Autodesk Inventor part; units mm, degrees
ref_plane "YZ Plane" through (0, 0, 0) normal (1, 0, 0) x (0, 1, 0)
ref_plane "XZ Plane" through (0, 0, 0) normal (0, 1, 0) x (-1, 0, 0)
ref_plane "XY Plane" through (0, 0, 0) normal (0, 0, 1) x (1, 0, 0)
sketch "Sketch1" plane through (0, 0, 0) normal (0, 1, 0) x (-1, 0, 0)
  line L0 (120, 102) -> (90, 102)
  line L1 (120, -102) -> (90, -102)
  line L2 (120, 102) -> (120, -102)
  line L3 (90, 102) -> (90, 50)
  line L4 (90, -50) -> (90, -102)
  line L5 (90, 50) -> (15, 50)
  line L6 (90, -50) -> (15, -50)
  line L7 (15, 50) -> (15, 102)
  line L8 (15, -50) -> (15, -102)
  line L9 (15, 102) -> (-15, 102)
  line L10 (15, -102) -> (-15, -102)
  line L11 (-15, 102) -> (-15, 50)
  line L12 (-15, -50) -> (-15, -102)
  line L13 (-15, 50) -> (-90, 50)
  line L14 (-15, -50) -> (-90, -50)
  line L15 (-90, 50) -> (-90, 102)
  line L16 (-90, -50) -> (-90, -102)
  line L17 (-90, 102) -> (-120, 102)
  line L18 (-90, -102) -> (-120, -102)
  line L19 (-120, 102) -> (-120, -102)
  line L20 (120, 0) -> (-120, 0) construction
  line L21 (0, 102) -> (0, -102) construction
  point P0 (0, 0)
  point P1 (0, 0)
  dimension "d0" = 204
  dimension "d1" = 30
  dimension "d3" = 75
  dimension "d4" = 52
  dimension "d5" = 100
extrude "Extrusion1" add sketch "Sketch1" along normal blind 5
sketch "Sketch2" plane through (0, 5, 0) normal (0, 1, 0) x (1, 0, 0)
  line L0 (-115, -90.5) -> (-95, -90.5)
  line L1 (-95, -90.5) -> (-95, -50)
  line L2 (-95, -50) -> (-115, -50)
  line L3 (-115, -50) -> (-115, -90.5)
  line L4 (-120, -102) -> (-90, -102)
  line L5 (-120, 102) -> (-120, -102)
  line L6 (-90, -102) -> (-90, -50)
  line L7 (-10, -90.5) -> (10, -90.5)
  line L8 (10, -90.5) -> (10, -50)
  line L9 (10, -50) -> (-10, -50)
  line L10 (-10, -50) -> (-10, -90.5)
  line L11 (95, -90.5) -> (115, -90.5)
  line L12 (115, -90.5) -> (115, -50)
  line L13 (115, -50) -> (95, -50)
  line L14 (95, -50) -> (95, -90.5)
  line L15 (-15, -50) -> (-15, -102)
  line L16 (90, -50) -> (90, -102)
  line L17 (-115, 50) -> (-95, 50)
  line L18 (-95, 50) -> (-95, 90.5)
  line L19 (-95, 90.5) -> (-115, 90.5)
  line L20 (-115, 90.5) -> (-115, 50)
  line L21 (-10, 50) -> (10, 50)
  line L22 (10, 50) -> (10, 90.5)
  line L23 (10, 90.5) -> (-10, 90.5)
  line L24 (-10, 90.5) -> (-10, 50)
  line L25 (95, 50) -> (115, 50)
  line L26 (115, 50) -> (115, 90.5)
  line L27 (115, 90.5) -> (95, 90.5)
  line L28 (95, 90.5) -> (95, 50)
  line L29 (-90, 102) -> (-120, 102)
  line L30 (-90, 50) -> (-90, 102)
  line L31 (-15, 102) -> (-15, 50)
  line L32 (90, 102) -> (90, 50)
  point P0 (0, 0)
  point P1 (-105, 50)
  point P2 (0, 50)
  point P3 (105, 50)
  point P4 (105, 90.5)
  point P5 (0, 90.5)
  point P6 (-105, 90.5)
  dimension "d8" = 11.5
  dimension "d9" = 5
  dimension "d10" = 5
  dimension "d11" = 40.5
  dimension "d12" = 5
  dimension "d13" = 5
  dimension "d14" = 5
  dimension "d15" = 11.5
  dimension "d16" = 5
  dimension "d17" = 40.5
  dimension "d18" = 5
  dimension "d19" = 5
extrude "Extrusion2" cut sketch "Sketch2" against normal up to next
equation "\"d1\" = s_depth + 2 * b_mat_thickness"
equation "\"d3\" = b_leg_space"
equation "\"d4\" = s_land + s_width + b_mat_thickness"
equation "\"d5\" = b_core_width"
equation "\"d6\" = b_mat_thickness"
equation "\"d8\" = b_mat_thickness + s_land"
equation "\"d9\" = b_mat_thickness"
equation "\"d10\" = b_mat_thickness"
equation "\"d11\" = s_width"
equation "\"d12\" = b_mat_thickness"
equation "\"d13\" = b_mat_thickness"
equation "\"d14\" = b_mat_thickness"
equation "\"d15\" = d8"
equation "\"d16\" = b_mat_thickness"
equation "\"d17\" = s_width"
equation "\"d18\" = b_mat_thickness"
equation "\"d19\" = b_mat_thickness"
equation "\"d20\" = 0.5 * b_mat_thickness"
properties part number "Body_bottom"
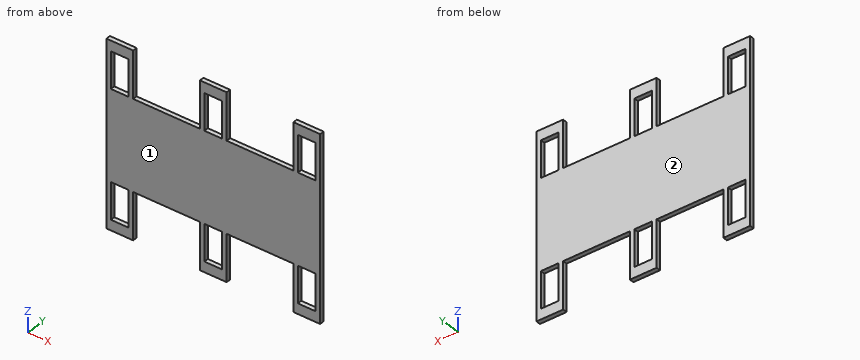
Could you check a few things on this model? Use its own coordinates, in mm. Face numbers are marked on the shaded views. Give positions to 0.01 mm unless a question says otherwise; leave off trailing zeros. Order: outer loops, then holes, each group sorted by start corner. A loop starts at its lowest first (then second) coordinate and runs counter-clockwise, first axis right, second up. Notation, with made-up numbers: (-27.5, 70) - (13.5, 70) arc R12 ccw to (13.5, 92) - close; hole circle Ø9 at (74, 47). An arc over 180 degrees is marked (long way). Return JSON: item names as keys, results as strings. Group by question number.
Q1. Suppose I cut it at D-D, the plane x = 60.5. Please give me the cut outline in (y, z), and give its area (3 significant figures).
Q2. Thinking about a two-plate mould opening in Y: for the marked faces 1 and 2, which applies, pulls with the +Y half, pulls with the -Y half, needs draft (parallel to the pull), parting line crosses it, or undercut?
Q3. Suppose I cut it at A-A, the plane x = -6. Please give me the cut outline in (y, z).
Q4. Suppose I cut it at C-C, the plane y = 3.4. State how many separate pieces and enclosed holes the cut face has, and give its area (3 significant figures).
Q5. Will this pin go through, and if not, where does the flat tip stop? pin 1 Ø1.5 at (x, y) = (-47, 3.5) entering from -Z.
Q6. Please list where these lines run through material, in increasing order: line 1 along X through (y, z) = (2.25, 67); line 2 along Z through (x, y) = (106.5, 4); line 3 along Z through (x, y) = (-65.5, 3.15). Write a range as [from, to].
Q7. Suppose I cut it at B-B, the plane z = -78. Please give me the cut outline in (x, y), and give its area (3 significant figures).
Resolved:
{
 "1": {"outline": "(0, -50) - (5, -50) - (5, 50) - (0, 50) - close", "area": "500 mm2"},
 "2": {"face 1": "pulls with the -Y half", "face 2": "pulls with the +Y half"},
 "3": {"outline": "(0, -102) - (5, -102) - (5, -90.5) - (0, -90.5) - close; (0, -50) - (5, -50) - (5, 50) - (0, 50) - close; (0, 90.5) - (5, 90.5) - (5, 102) - (0, 102) - close"},
 "4": {"separate pieces": "1", "enclosed holes": "6", "area": "28,500 mm2"},
 "5": {"pin 1": "stops at z = -50"},
 "6": {"line 1": "x = [-120, -115], [-95, -90], [-15, -10], [10, 15], [90, 95], [115, 120]", "line 2": "z = [-102, -90.5], [-50, 50], [90.5, 102]", "line 3": "z = [-50, 50]"},
 "7": {"outline": "(-120, 0) - (-115, 0) - (-115, 5) - (-120, 5) - close; (-95, 0) - (-90, 0) - (-90, 5) - (-95, 5) - close; (-15, 0) - (-10, 0) - (-10, 5) - (-15, 5) - close; (10, 0) - (15, 0) - (15, 5) - (10, 5) - close; (90, 0) - (95, 0) - (95, 5) - (90, 5) - close; (115, 0) - (120, 0) - (120, 5) - (115, 5) - close", "area": "150 mm2"}
}
